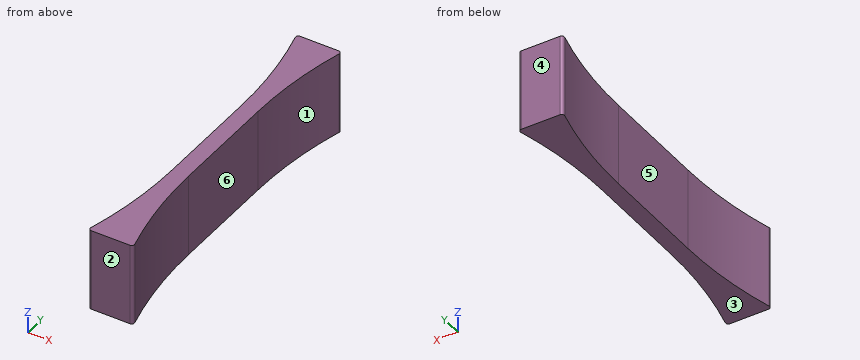
from build123d import *

# Parameters (mm, degrees)
BOSS_EXTRUDE1_DEPTH = 15
FILLET1_R           = 0.5


with BuildPart() as part:
    # Sketch1 → Boss-Extrude1 (new body)
    with BuildSketch(Plane.XY):
        with BuildLine():
            Line((0, 0), (1.5, 0))
            Line((1.5, 0), (1.5, 10))
            ThreePointArc((1.5, 10), (2.172674131, 20.089300148), (4.178788881, 30))
            Line((4.178788881, 30), (0, 30))
            Line((0, 30), (0, 0))
        make_face()
    boss_extrude1 = extrude(amount=BOSS_EXTRUDE1_DEPTH)

    # Mirror1: Boss-Extrude1 across plane
    add(boss_extrude1.mirror(Plane(origin=(0, 30, 15), x_dir=(0, 0, 1), z_dir=(1, 0, 0))))

    # Mirror6: part across plane


with BuildPart() as part_1:
    add(part.part)
    add(part.part.mirror(Plane(origin=(0, 0, 15), x_dir=(0, 0, 1), z_dir=(0, 1, 0))))

    # Fillet1
    fillet1_edges = [part_1.edges().sort_by_distance(p)[0] for p in [
        (-4.178788881, 30, 7.5),
        (4.178788881, -30, 7.5),
        (-4.178788881, -30, 7.5),
        (4.178788881, 30, 7.5),
    ]]
    fillet(fillet1_edges, radius=FILLET1_R)


solid = part_1.part
Geometry: final body of the model. Coordinates: model frame, mm. Face numbers are marked on the shaded views. A direction names the side the tool comes from. Give positions to 0.01 mm unless a question says otherwise; leave off trailing zeros. Write each loop counter-clockwise with the first axis right and the second up, starting at its lowest first coordinate (ties: lowest second). Pieces come first, ordered by that corner, then holes. Notation, with made-up numbers: (64.5, 9.25) - (116.5, 9.25) arc R31 cw to (116.5, 36.25) - close; hole circle Ø3 at (21, 61). An arc over 180 degrees is marked (long way). Return JSON: item names as keys, results as strings. Group by question number.
1) Line query: line 1 (X direction, y = -3, z = 10.5); line 2 (X direction, y = -25, z = 8.5). Output: solid intervals per line, ascending.
2) Set-up query: the marked faces 4, 5 and 6. Return all of +Z, -Z, +X, -X, +Y, -Y with unobstructed straight access to the full face (end or side cutting, diameter ignored); none if empty.
3) First-contact query: P1, Ø4.5, axis at y = 5, z = 11, coming from the -X side; P2, Ø7.5, axis at y = 2.5, z = 9, coming from the +X side. Flat tips, straight axial feed; report the tip coordinate or a pass-through.
4) Mould query, pull axis Y, two halves, no side actions, for the marked faces 1, 2 and 3. Classes: released by +Y, released by -Y, zero draft, split by the parting line, or undercut.
5) Section B-B on z = 2. Return the cut outline in (x, y), plus the area to 3 significant figures.
Filled in:
{
 "1": {"line 1": "x = -1.5 to 1.5", "line 2": "x = -2.99 to 2.99"},
 "2": {"face 4": "+Z, -Z, +X, -X, +Y", "face 5": "+Z, -Z, -X", "face 6": "+Z, -Z, +X"},
 "3": {"P1": "stops at x = -1.5", "P2": "stops at x = 1.5"},
 "4": {"face 1": "undercut", "face 2": "released by -Y", "face 3": "zero draft"},
 "5": {"outline": "(-4.01, -29.37) arc R0.5 ccw to (-3.53, -30) - (3.53, -30) arc R0.5 ccw to (4.01, -29.37) arc R76 cw to (1.5, -10) - (1.5, 10) arc R76 cw to (4.01, 29.37) arc R0.5 ccw to (3.53, 30) - (-3.53, 30) arc R0.5 ccw to (-4.01, 29.37) arc R76 cw to (-1.5, 10) - (-1.5, -10) arc R76 cw to start", "area": "251 mm^2"}
}
